The listing builds one solid part. Answer for the finished solid, in the listing's coordinates (mm). Face numbers are marked on the shaded views. Give positions to 0.01 mm unless a question says otherwise; leave off trailing zeros. Loops run counter-clockwise (first coordinate to the right, second up) from the corner with the lowest first, then second, coordinate; pieces in that order, holes last. Notation, with made-up numbers: M 75,6 L 120,6 A24 ccw 120,35 Z; hole C 68,44 d8. An arc over 180 degrees is marked long. Return JSON: item names as keys, results as strings.
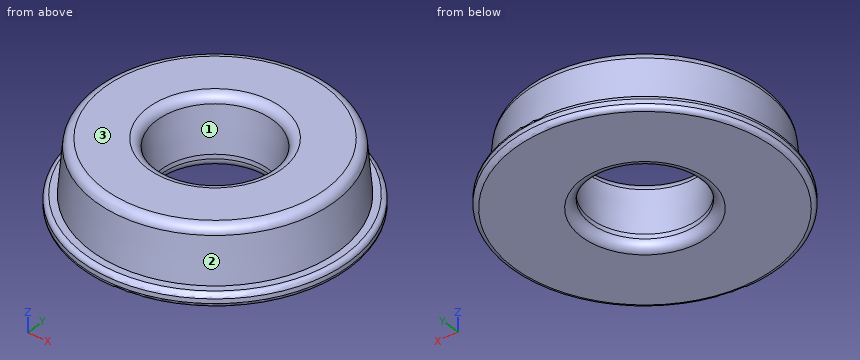
from build123d import *

# Parameters (mm, degrees)
F0_R     = 27.5
F0_R_2   = 12
F1_DEPTH = 12
F1_TAPER = 5
F2_R     = 30
F2_R_2   = 12
F3_DEPTH = 3
F4_R     = 2
F5_R     = 1


with BuildPart() as f1:
    # F0 (on Top) → F1 (new body)
    with BuildSketch(Plane.XY):
        Circle(F0_R)
        Circle(F0_R_2, mode=Mode.SUBTRACT)
    extrude(amount=F1_DEPTH, taper=F1_TAPER)

    # F2 (on Top) → F3 (join)
    with BuildSketch(Plane.XY):
        Circle(F2_R)
        Circle(F2_R_2, mode=Mode.SUBTRACT)
    extrude(amount=-F3_DEPTH)

    # F4
    f4_edges = [f1.edges().sort_by_distance(p)[0] for p in [
        (-26.450136, 0, 12),
        (-12, 0, -3),
        (-13.049864, 0, 12),
    ]]
    fillet(f4_edges, radius=F4_R)

    # F5
    f5_edges = [f1.edges().sort_by_distance(p)[0] for p in [
        (-30, 0, -3),
        (-30, 0, 0),
    ]]
    fillet(f5_edges, radius=F5_R)


solid = f1.part
(1) The part is cut by section A-A (x = 0). Determine the outline of the cut face in (y, z), and give its area (3 significant figures).
Values follow:
{"outline": "M -30,-2 A1 ccw -29,-3 L -14,-3 A2 ccw -12,-1 L -12,0 L -12.89,10.17 A2 ccw -14.88,12 L -24.62,12 A2 ccw -26.61,10.17 L -27.5,0 L -29,0 A1 ccw -30,-1 Z; M 12,-1 A2 ccw 14,-3 L 29,-3 A1 ccw 30,-2 L 30,-1 A1 ccw 29,0 L 27.5,0 L 26.61,10.17 A2 ccw 24.62,12 L 14.88,12 A2 ccw 12.89,10.17 L 12,0 Z", "area": "449 mm²"}
(2) Straight lines are drawn through the part: line 1 along Y through (x, z) = (0, -0.7); line 2 along Y through (x, z) = (0, -0.25); line 3 along X through (y, z) = (-11, 9.25). For each, find the intervals that lie inside material, in ascending order.
Values follow:
{"line 1": "-29.95 to -12, 12 to 29.95", "line 2": "-29.66 to -12, 12 to 29.66", "line 3": "-24.32 to -6.56, 6.56 to 24.32"}
(3) Given pin 1 (8 mm diameter, centred on x = -17, z = 2, fed in from -Y); pin 2 (4 mm diameter, centred on y = 12, z = 3.5, fed in from +X); pin 3 (1.5 mm diameter, centred on y = 13, z = 0, fed in from -X); pin 4 (14.5 mm diameter, centred on x = 0, y = 0, fed in from +Z), each flat-ended and moving along its own axis, determine where each tip first touches the part or whether it passes through.
Values follow:
{"pin 1": "y = -26.46", "pin 2": "x = 25.31", "pin 3": "x = -27.16", "pin 4": "through"}
(4) The part is cut by section B-B (z = 8.75). Determine the outline of the cut face in (x, y).
Values follow:
{"outline": "C 0,0 d53.47; hole C 0,0 d25.53"}
(5) Determine the mould class of the marked faces 1, 2 and 3 for opening direction X: released by +X, released by -X, zero draft, split by the parting line, or undercut.
Values follow:
{"face 1": "undercut", "face 2": "split by the parting line", "face 3": "zero draft"}
(6) The part is cut by section C-C (z = 2). Determine the outline of the cut face in (x, y).
Values follow:
{"outline": "C 0,0 d54.65; hole C 0,0 d24.35"}
